The model under review builds one solid part; all positions refer to its coordinate system, in mm. Face numbers are marked on the shaded views. A direction names the side the tool comes from. Round coordinates to 2 decimals unless told otherwise and drop trailing zeros. Write each loop counter-clockwise with the first axis right and the second up, starting at its lowest first coordinate (ties: lowest second). Pieces come first, ordered by that corner, then holes. Notation, with made-up numbers: M 83,12.25 L 89,12.25 A14 cw 89,31.25 Z; hole C 22.25,11.5 d10. An arc over 180 degrees is marked long. One line per item, written item: value. Start each with the question number.
1) Take a section at A-A, the plane x = 0. Write out the cut boundary in (y, z), and give its area (3 significant figures).
2) Take a section at C-C, the plane y = 63. Write out the cut boundary in (x, z).
3) Wall thickness on probe 1 along Y at (x, z) = (-7.5, 74.5); probe 2 along Z at (x, y) = (-15, 55); probe 3 along Z at (x, y) = (11, 107.5): over which ranges is each line inside the solid? List them lowest first.
4) For P1, Ø5, axis at x = 2, y = 198.5, coming from the +Z side; P2, Ø20.5, axis at y = 138, z = 19.5, coming from the -X side; P3, Ø1, axis at x = 8.5, z = 41, coming from the +Y side; P4, Ø12, axis at x = -3.5, y = 170.5, coming from the -Z side, all flat-tipped, find the tip position at first contact; note any pin that passes through.
5) Tool access review of the marked faces 1, 2 and 3: name each direction out of +Z, -Z, +X, -X, +Y, -Y from which nothing blocks a thin tool from reaching the whole face with its end or side.
6) Take a section at B-B, the plane y = 147. Write out the cut boundary in (x, z), and give its area (3 significant figures).
from build123d import *

# Parameters (mm, degrees)
SKETCH1_R                  = 5.25
EXTRUDE1_DEPTH             = 6
PROCESS_BENDS1_START       = -28
PROCESS_BENDS1_DEPTH       = 56
PROCESS_BENDS1_START_2     = -20
PROCESS_BENDS1_2_DEPTH     = 40
PROCESS_BENDS1_START_3     = -27.5
PROCESS_BENDS1_3_DEPTH     = 55
PROCESS_BENDS1_START_4     = 67
PROCESS_BENDS1_4_DEPTH     = 8
PROCESS_BENDS1_START_5     = 49.934347195
PROCESS_BENDS1_5_OUTLINE_R = 5.25
PROCESS_BENDS1_5_DEPTH     = 43.065652805
CHAMFER1_SIZE              = 4.75


with BuildPart() as part:
    # Sketch1 → Extrude1 (new body)
    with BuildSketch(Plane.XY):
        with BuildLine():
            Line((-15, 0), (15, 0))
            ThreePointArc((15, 0), (25.542393073, 5.783754896), (26.328847338, 17.782728272))
            Line((26.328847338, 17.782728272), (20.93692213, 29.345749196))
            ThreePointArc((20.93692213, 29.345749196), (20.237039929, 31.407535674), (20, 33.571931813))
            Line((20, 33.571931813), (20, 266.5))
            ThreePointArc((20, 266.5), (19.707106781, 267.207106781), (19, 267.5))
            Line((19, 267.5), (-19, 267.5))
            ThreePointArc((-19, 267.5), (-19.707106781, 267.207106781), (-20, 266.5))
            Line((-20, 266.5), (-20, 33.571931813))
            ThreePointArc((-20, 33.571931813), (-20.237039929, 31.407535674), (-20.93692213, 29.345749196))
            Line((-20.93692213, 29.345749196), (-26.328847338, 17.782728272))
            ThreePointArc((-26.328847338, 17.782728272), (-25.542393073, 5.783754896), (-15, 0))
        make_face()
        with Locations((15, 12.5)):
            Circle(SKETCH1_R, mode=Mode.SUBTRACT)
        with Locations(Location((-15, 12.5, 0), (0, 0, 180))):
            Circle(SKETCH1_R, mode=Mode.SUBTRACT)
    extrude(amount=EXTRUDE1_DEPTH)

    # Process-Bends1: read off the stored shape, not the designer's step
    # Process-Bends1 outline → Process-Bends1 (cut)
    with BuildSketch(Plane.YZ.offset(PROCESS_BENDS1_START)):
        with BuildLine():
            Line((202.708327384, 5.276311449), (217.204873948, 0))
            Line((217.204873948, 0), (267.5, 0))
            Line((267.5, 0), (267.5, 6))
            Line((267.5, 6), (198.604085664, 6))
            ThreePointArc((198.604085664, 6), (200.687863796, 5.817693036), (202.708327384, 5.276311449))
        make_face()
        with BuildLine():
            Line((0, 0), (92.140807255, 0))
            ThreePointArc((92.140807255, 0), (87.548606067, 0.91344561), (83.655525881, 3.514718626))
            Line((83.655525881, 3.514718626), (81.170244507, 6))
            Line((81.170244507, 6), (0, 6))
            Line((0, 6), (0, 0))
        make_face()
    extrude(amount=PROCESS_BENDS1_DEPTH, mode=Mode.SUBTRACT)

    # Process-Bends1 2 outline → Process-Bends1 2 (add)
    with BuildSketch(Plane.YZ.offset(PROCESS_BENDS1_START_2)):
        with BuildLine():
            Line((262.773728027, -22.970773129), (264.825848887, -17.332617404))
            Line((264.825848887, -17.332617404), (217.204873948, 0))
            Line((217.204873948, 0), (198.604085664, 0))
            ThreePointArc((198.604085664, 0), (199.64597473, -0.091153482), (200.656206524, -0.361844275))
            Line((200.656206524, -0.361844275), (262.773728027, -22.970773129))
        make_face()
        with BuildLine():
            Line((81.170244507, 6), (92.140807255, 6))
            ThreePointArc((92.140807255, 6), (89.844706661, 6.456722805), (87.898166568, 7.757359313))
            Line((87.898166568, 7.757359313), (57.691706508, 37.963819374))
            ThreePointArc((57.691706508, 37.963819374), (56.39107, 39.910359467), (55.934347195, 42.206460061))
            Line((55.934347195, 42.206460061), (55.934347195, 79.065652805))
            Line((55.934347195, 79.065652805), (49.934347195, 79.065652805))
            Line((49.934347195, 79.065652805), (49.934347195, 42.206460061))
            ThreePointArc((49.934347195, 42.206460061), (50.847792805, 37.614258872), (53.44906582, 33.721178686))
            Line((53.44906582, 33.721178686), (81.170244507, 6))
        make_face()
    extrude(amount=PROCESS_BENDS1_2_DEPTH)

    # Process-Bends1 3 outline → Process-Bends1 3 (add)
    with BuildSketch(Plane.YZ.offset(PROCESS_BENDS1_START_3)):
        with BuildLine():
            Line((81.170244507, 6), (92.140807255, 6))
            ThreePointArc((92.140807255, 6), (89.844706661, 6.456722805), (87.898166568, 7.757359313))
            Line((87.898166568, 7.757359313), (57.691706508, 37.963819374))
            ThreePointArc((57.691706508, 37.963819374), (56.39107, 39.910359467), (55.934347195, 42.206460061))
            Line((55.934347195, 42.206460061), (55.934347195, 79.065652805))
            Line((55.934347195, 79.065652805), (49.934347195, 79.065652805))
            Line((49.934347195, 79.065652805), (49.934347195, 42.206460061))
            ThreePointArc((49.934347195, 42.206460061), (50.847792805, 37.614258872), (53.44906582, 33.721178686))
            Line((53.44906582, 33.721178686), (81.170244507, 6))
        make_face()
    extrude(amount=PROCESS_BENDS1_3_DEPTH)

    # Process-Bends1 4 outline → Process-Bends1 4 (cut)
    with BuildSketch(Plane(origin=(0, 0, 0), x_dir=(1, 0, 0), z_dir=(0, 0.3420201433256691, 0.9396926207859083)).offset(PROCESS_BENDS1_START_4)):
        with BuildLine():
            Line((20, 254.783000281), (19, 254.783000281))
            ThreePointArc((19, 254.783000281), (19.707106781, 254.490107062), (20, 253.783000281))
            Line((20, 253.783000281), (20, 254.783000281))
        make_face()
        with BuildLine():
            ThreePointArc((-20, 253.783000281), (-19.707106781, 254.490107062), (-19, 254.783000281))
            Line((-19, 254.783000281), (-20, 254.783000281))
            Line((-20, 254.783000281), (-20, 253.783000281))
        make_face()
    extrude(amount=PROCESS_BENDS1_4_DEPTH, mode=Mode.SUBTRACT)

    # Process-Bends1 5 outline → Process-Bends1 5 (cut)
    with BuildSketch(Plane(origin=(0, 0, 0), x_dir=(1, 0, 0), z_dir=(0, 1, 0)).offset(PROCESS_BENDS1_START_5)):
        with BuildLine():
            ThreePointArc((-20.93692213, -49.719903609), (-20.237039929, -47.658117131), (-20, -45.493720992))
            Line((-20, -45.493720992), (-20, -6))
            Line((-20, -6), (-27.5, -6))
            Line((-27.5, -6), (-27.5, -66.565652806))
            ThreePointArc((-27.5, -66.565652806), (-27.203700089, -63.860157632), (-26.328847338, -61.282924534))
            Line((-26.328847338, -61.282924534), (-20.93692213, -49.719903609))
        make_face()
        with BuildLine():
            ThreePointArc((26.328847338, -61.282924534), (27.203700089, -63.860157632), (27.5, -66.565652806))
            Line((27.5, -66.565652806), (27.5, -6))
            Line((27.5, -6), (20, -6))
            Line((20, -6), (20, -45.493720992))
            ThreePointArc((20, -45.493720992), (20.237039929, -47.658117131), (20.93692213, -49.719903609))
            Line((20.93692213, -49.719903609), (26.328847338, -61.282924534))
        make_face()
        with BuildLine():
            ThreePointArc((27.5, -66.565652806), (23.838834765, -75.404487571), (15, -79.065652805))
            Line((15, -79.065652805), (27.5, -79.065652805))
            Line((27.5, -79.065652805), (27.5, -66.565652806))
        make_face()
        with BuildLine():
            ThreePointArc((-15, -79.065652805), (-23.838834765, -75.404487571), (-27.5, -66.565652806))
            Line((-27.5, -66.565652806), (-27.5, -79.065652805))
            Line((-27.5, -79.065652805), (-15, -79.065652805))
        make_face()
        with Locations((-15, -66.565652805)):
            Circle(PROCESS_BENDS1_5_OUTLINE_R)
        with Locations((15, -66.565652805)):
            Circle(PROCESS_BENDS1_5_OUTLINE_R)
    extrude(amount=PROCESS_BENDS1_5_DEPTH, mode=Mode.SUBTRACT)

    # Chamfer1
    chamfer1_edges = [part.edges().sort_by_distance(p)[0] for p in [
        (9.75, 49.934347195, 66.565652805),
        (-20.25, 49.934347195, 66.565652805),
    ]]
    chamfer(chamfer1_edges, length=CHAMFER1_SIZE)


solid = part.part
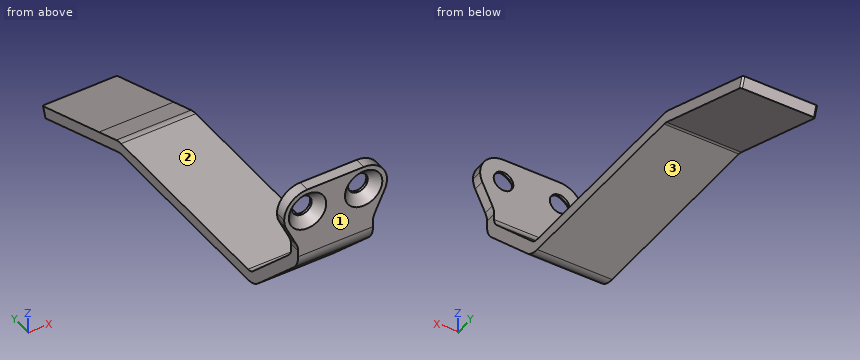
Checked values:
1. outline: M 49.93,42.21 A12 ccw 53.45,33.72 L 83.66,3.51 A12 ccw 92.14,0 L 198.6,0 A6 cw 200.66,-0.36 L 262.77,-22.97 L 264.83,-17.33 L 202.71,5.28 A12 ccw 198.6,6 L 92.14,6 A6 cw 87.9,7.76 L 57.69,37.96 A6 cw 55.93,42.21 L 55.93,79.07 L 49.93,79.07 Z
1. area: 1,620 mm2
2. outline: M -20,24.17 L 20,24.17 L 20,32.66 L -20,32.66 Z
3. probe 1: y = 49.93 to 55.93
3. probe 2: z = 32.17 to 61.32, 71.82 to 79.07
3. probe 3: z = 0 to 6
4. P1: stops at z = 6
4. P2: passes through
4. P3: stops at y = 56.18
4. P4: stops at z = 0
5. face 1: +Z, -Z, +X, -X, -Y
5. face 2: +Z, +X, -X, +Y
5. face 3: -Z, +X, -X, -Y
6. outline: M -20,0 L 20,0 L 20,6 L -20,6 Z
6. area: 240 mm2
